Autodesk Inventor part; units mm, degrees
ref_plane "Work Plane1" through (0, 15, 0) normal (0, 1, 0) x (-1, 0, 0)
ref_plane "YZ Plane" through (0, 0, 0) normal (1, 0, 0) x (0, 1, 0)
ref_plane "XY Plane" through (0, 0, 0) normal (0, 0, 1) x (1, 0, 0)
ref_plane "Work Plane1" through (0, 15, 0) normal (0, 1, 0) x (-1, 0, 0)
sketch "Sketch1" plane through (0, 0, 0) normal (0, 0, 1) x (1, 0, 0)
  line L0 (0, 0) -> (0, 20)
  line L1 (0, 0) -> (20, 0)
  arc A0 (20, 0) -> (0, 20) centre (0, 0) ccw
  line L2 (0, -4.8284) -> (0, 28.9706)
  dimension "d2" = 20
revolve "Revolution1" add sketch "Sketch1" angle 360 about axis through (0, -10, 0) along (0, 1, 0)
sketch "Sketch2" plane through (0, 15, 0) normal (0, 1, 0) x (-1, 0, 0)
  point P0 (0, 0)
  point P1 (0, 0)
hole "Hole1" at (0, 15, 0) direction (0, -1, 0) diameter 4.5 end through all counterbore diameter 8 counterbore depth 4
shell "Shell1" thickness 2 removed faces 1 at (13.8841, 0, 1.6858)
sketch "Sketch3" plane through (0, 0, 0) normal (0, -1, 0) x (1, 0, 0)
  circle A0 centre (0, 0) radius 4.25
  circle A1 centre (0, 0) radius 2.25
extrude "Extrusion1" cut sketch "Sketch3" against normal blind 9
properties part number "Ball_Upper Half" material "Nylon 6/6"
CAD build for the part. Positions are in the model's coordinates, mm. A direction names the side the tool comes from. Coordinates: 2 decimals unless noted, no trailing zeros. Write each loop counter-clockwise with the first axis right and the second up, starting at its lowest first coordinate (ties: lowest second). Pieces come first, ordered by that corner, then holes.
(1) Cut at D-D, the plane y = 12.75. List the corners of the cut face in (x, z), and give its area (3 significant figures).
(2) 3-axis set-ups, long thin cutter, end or side, ignore diameter. For faces 1 (the face through (0, 9, 3)), 2 (the face through (3.905, 12.972, -0.867)): which of +Z, -Z, +X, -X, +Y, -Y reach the whole face in a straight line?
(3) Flat gauge pins, fed straight in: pin 1 (5 mm diameter, centred on x = 10.5, y = 17.5, fed in from +Z); pin 2 (6 mm diameter, centred on x = 2.5, z = 2.5, fed in from +Y); pin 3 (1 mm diameter, centred on y = 4, z = -9.5, fed in from -X). Where does each tip first touch, or does it go through?
(4) Cut at B-B, the plane z = -1. List the corners of the cut face in (x, y).
(5) Cut at A-A, the plane x = -5. List the corners of the cut face in (y, z).
(6) Two-plate mould, pull along Z, no slides. Class faces 3 (the face through (2, 11, 2)), 4 (the face through (18, 0, -3)): +Z half, -Z half, draft (parallel to the pull), parting line (faces both ways), or undercut.
(7) Cut at C-C, the plane y = 16.25. List the corners of the cut face in (x, z).
(8) Drill centre lines: probe 1 along X at (y, z) = (10.25, -3); probe 2 along Z at (x, y) = (0, 10.4); probe 3 along Z at (x, y) = (0, 9.55). Where is each one in solid material? Low to high.
Geometry says:
1. outline: circle Ø30.82 at (0, 0); circle Ø12 at (0, 0); hole circle Ø25.41 at (0, 0); hole circle Ø8 at (0, 0)
1. area: 302 mm2
2. face 1: -Y
2. face 2: none
3. pin 1: stops at z = 8.9
3. pin 2: stops at y = 19.99
3. pin 3: stops at x = -17.43
4. outline: (-19.97, 0) - (-17.97, 0) arc R17.97 cw to (-5.92, 16.97) - (-5.92, 9) - (-2.02, 9) - (-2.02, 11) - (-3.87, 11) - (-3.87, 15) - (3.87, 15) - (3.87, 11) - (2.02, 11) - (2.02, 9) - (5.92, 9) - (5.92, 16.97) arc R17.97 cw to (17.97, 0) - (19.97, 0) arc R19.97 ccw to start; hole (-5.83, 17) - (5.83, 17) arc R17.97 ccw to start
5. outline: (0, -19.36) arc R19.36 ccw to (0, 19.36) - (0, 17.29) arc R17.29 cw to (16.97, 3.32) - (9, 3.32) - (9, -3.32) - (16.97, -3.32) arc R17.29 cw to (0, -17.29) - close; hole (17, -3.16) arc R17.29 ccw to (17, 3.16) - close
6. face 3: undercut
6. face 4: draft
7. outline: circle Ø23.32 at (0, 0); circle Ø12 at (0, 0); hole circle Ø15.48 at (0, 0)
8. probe 1: x = -16.91 to -14.49, -5.2 to 5.2, 14.49 to 16.91
8. probe 2: z = -17.08 to -14.69, -6 to -2.25, 2.25 to 6, 14.69 to 17.08
8. probe 3: z = -17.57 to -15.26, -6 to -2.25, 2.25 to 6, 15.26 to 17.57
